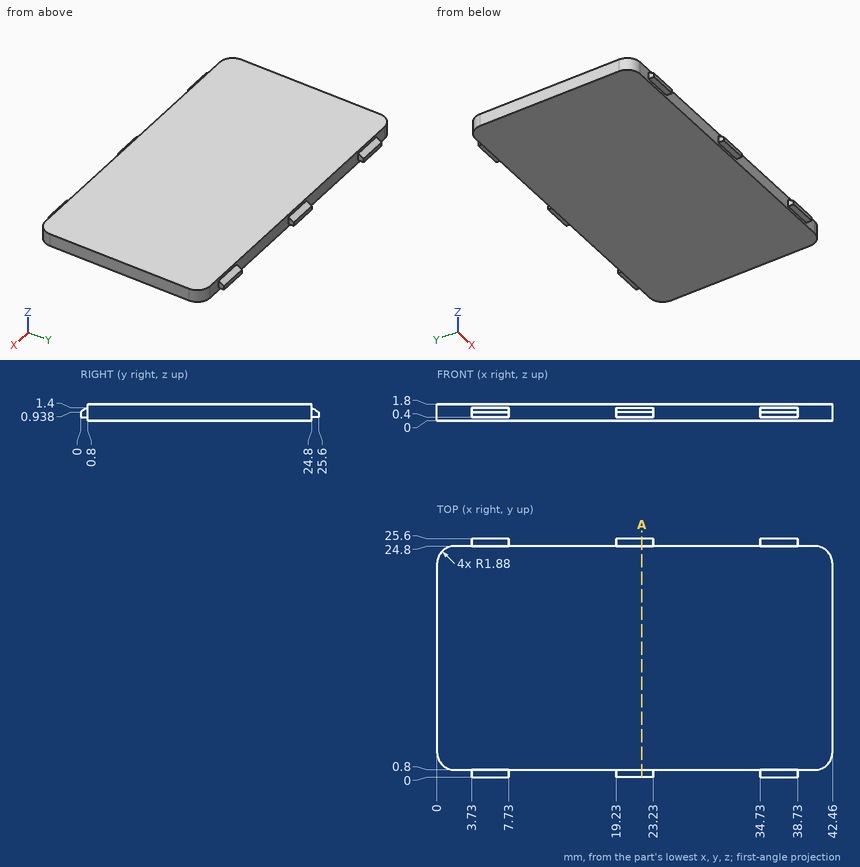
Check sheet for the drawn part. Datum: minimum x, y, z corner. Units: mm. Round coordinates to 2 decimals unless told otherwise and drop trailing zeros. Order: outer loops, then holes, each group sorted by start corner. A loop starts at its lowest first (then second) coordinate and runs counter-clockwise, first axis right, second up.
1) Go/stop test with a flat-tipped pin: pin 1 Ø0.6 at (y, z) = (25.5, 1) entering from +X. Record where the tip stops, or that it passes through.
2) Scan lines: line 1 (Y direction, x = 19, z = 1.5); line 2 (X direction, y = 2, z = 0.35); line 3 (Y direction, x = 22, z = 1.05). Record each from-to range of solid material in increasing order.
3) Section check A-A (x = 22). Record the boundary of the cut face in (y, z).
Result:
1. pin 1: stops at x = 38.73
2. line 1: y = 0.8 to 24.8
2. line 2: x = 0.13 to 42.33
2. line 3: y = 0.19 to 25.41
3. outline: (0, 0.4) - (0.8, 0.4) - (0.8, 0) - (24.8, 0) - (24.8, 0.4) - (25.6, 0.4) - (25.6, 0.94) - (24.8, 1.4) - (24.8, 1.8) - (0.8, 1.8) - (0.8, 1.4) - (0, 0.94) - close
